Autodesk Inventor part; units mm, degrees
ref_plane "YZ Plane" through (0, 0, 0) normal (1, 0, 0) x (0, 1, 0)
ref_plane "XZ Plane" through (0, 0, 0) normal (0, 1, 0) x (-1, 0, 0)
ref_plane "XY Plane" through (0, 0, 0) normal (0, 0, 1) x (1, 0, 0)
sketch "Sketch1" plane through (0, 0, 0) normal (0, 0, 1) x (1, 0, 0)
  line L0 (0, 0) -> (-140, 0)
  line L1 (-140, 0) -> (-140, 140)
  line L2 (-140, 140) -> (0, 140)
  line L3 (0, 140) -> (0, 0)
  circle A0 centre (-70, 70) radius 14.35
  line L4 (-130, 124.4) -> (-130, 130)
  line L5 (-10, 124.4) -> (-10, 130)
  line L6 (-10, 15.6) -> (-10, 10)
  line L7 (-130, 15.6) -> (-130, 10)
  line L8 (-140, 140) -> (-110, 140)
  line L9 (-110.0005, 135.0005) -> (-110.0005, 113.536)
  line L10 (-113.536, 110) -> (-135, 110)
  line L11 (-140, 110) -> (-140, 140)
  line L12 (-140, 0) -> (-110, 0)
  line L13 (-109.9998, 5.0002) -> (-109.9998, 26.4642)
  line L14 (-113.536, 30) -> (-135, 30)
  line L15 (-140, 30) -> (-140, 0)
  line L16 (0, 0) -> (-30, 0)
  line L17 (-30, 5.0002) -> (-30, 26.464)
  line L18 (-26.4645, 30) -> (-5, 30)
  line L19 (0, 30) -> (0, 0)
  line L20 (0, 140) -> (-30, 140)
  line L21 (-30, 135.0005) -> (-30, 113.536)
  line L22 (-26.4638, 110.0002) -> (-5, 110.0002)
  line L23 (0, 110) -> (0, 140)
  line L24 (-110.0005, 113.536) -> (-80.0116, 83.5551)
  line L25 (-56.4494, 59.9849) -> (-26.4645, 30)
  line L26 (-113.536, 110) -> (-83.5508, 80.0148)
  line L27 (-59.9852, 56.4492) -> (-30, 26.464)
  line L28 (-113.536, 30) -> (-83.5508, 59.9852)
  line L29 (-59.9861, 83.5534) -> (-29.9997, 113.5363)
  line L30 (-109.9998, 26.4642) -> (-80.0148, 56.4492)
  line L31 (-56.4492, 80.0148) -> (-26.4638, 110.0002)
  line L32 (-135, 110) -> (-135, 30)
  line L33 (-140, 30) -> (-140, 110)
  line L34 (-5, 110.0002) -> (-5, 30)
  line L35 (0, 30) -> (0, 110)
  line L36 (-110, 140) -> (-30, 140)
  line L37 (-30, 135.0005) -> (-110.0005, 135.0005)
  line L38 (-30, 0) -> (-110, 0)
  line L39 (-109.9998, 5.0002) -> (-30, 5.0002)
  arc A1 (-83.5508, 80.0148) -> (-83.5508, 59.9852) centre (-70, 70) ccw
  arc A2 (-59.9861, 83.5534) -> (-80.0116, 83.5551) centre (-70, 70) ccw
  arc A3 (-80.0148, 56.4492) -> (-59.9852, 56.4492) centre (-70, 70) ccw
  arc A4 (-56.4494, 59.9849) -> (-56.4492, 80.0148) centre (-70, 70) ccw
  line L40 (-130, 130) -> (-124.4, 130)
  line L41 (-124.4, 130) -> (-124.4, 119.4)
  line L42 (-124.4, 119.4) -> (-130, 119.4)
  line L43 (-130, 119.4) -> (-130, 130)
  line L44 (-130, 10) -> (-124.4, 10)
  line L45 (-124.4, 10) -> (-124.4, 20.6)
  line L46 (-124.4, 20.6) -> (-130, 20.6)
  line L47 (-130, 20.6) -> (-130, 10)
  line L48 (-10, 10) -> (-15.6, 10)
  line L49 (-15.6, 10) -> (-15.6, 20.6)
  line L50 (-15.6, 20.6) -> (-10, 20.6)
  line L51 (-10, 20.6) -> (-10, 10)
  line L52 (-10, 130) -> (-15.6, 130)
  line L53 (-15.6, 130) -> (-15.6, 119.4)
  line L54 (-15.6, 119.4) -> (-10, 119.4)
  line L55 (-10, 119.4) -> (-10, 130)
  line L56 (-113.536, 30) -> (-109.9998, 26.4642)
  line L57 (-30, 26.464) -> (-26.4645, 30)
  line L58 (-30, 113.536) -> (-26.4638, 110.0002)
  line L59 (-110.0005, 113.536) -> (-113.536, 110)
  point P0 (-110, 113.5355)
  point P1 (-110, 26.464)
  point P2 (-26.464, 110)
extrude "Extrusion2" add sketch "Sketch1" along normal blind 5 contours L0 L1 L2 L3 | L24 A2 L29 L58 L31 A4 L25 L57 L27 A3 L30 L56 L28 A1 L26 L59
properties part number "Joints_Remake_TestFit_V1"
Read the model definition and answer for the solid it produces. Units are mm, in the model's axes. Round coordinates to 2 decimals unless told otherwise and drop trailing zeros. Write each loop counter-clockwise with the first axis right and the second up, starting at its lowest first coordinate (ties: lowest second). Pieces come first, ordered by that corner, then holes.
1. The part is cut by section B-B, the plane y = 115.5. Determine the outline of the cut face in (x, z), then the cut area to 3 significant figures.
2. Determine the mould class of faces 1 (the face through (-15.6, 15, 2)), 2 (the face through (-69, 0, 2)) for opening direction Y: pulls with the +Y half, pulls with the -Y half, needs draft (parallel to the pull), parting line crosses it, or undercut.
3. Straight lines are drawn through the part: L1, parallel to Y at x = -70, z = 1.2; L2, parallel to X at y = 70.5, z = 3.7; L3, parallel to X at y = 104.5, z = 1.55. For each, find the intervals that lie inside material, in ascending order.
4. The part is cut by section C-C, the plane x = -70. Determine the outline of the cut face in (y, z).
5. The part is cut by section D-D, the plane z = 1.85. State how many separate pieces and enclosed holes the cut face has, then the cut area to 3 significant figures.
6. The part is cut by section A-A, the plane y = 70. Determine the outline of the cut face in (x, z), then the cut area to 3 significant figures.
Values:
1. outline: (-140, 0) - (-110, 0) - (-110, 5) - (-140, 5) - close; (-30, 0) - (0, 0) - (0, 5) - (-30, 5) - close
1. area: 300 mm2
2. face 1: undercut
2. face 2: pulls with the -Y half
3. L1: y = 0 to 5, 53.15 to 55.65, 84.35 to 86.85, 135 to 140
3. L2: x = -140 to -135, -86.84 to -84.34, -55.66 to -53.16, -5 to 0
3. L3: x = -140 to -135, -108.04 to -100.96, -39.04 to -31.96, -5 to 0
4. outline: (0, 0) - (5, 0) - (5, 5) - (0, 5) - close; (53.15, 0) - (55.65, 0) - (55.65, 5) - (53.15, 5) - close; (84.35, 0) - (86.85, 0) - (86.85, 5) - (84.35, 5) - close; (135, 0) - (140, 0) - (140, 5) - (135, 5) - close
5. separate pieces: 1
5. enclosed holes: 9
5. area: 6,030 mm2
6. outline: (-140, 0) - (-135, 0) - (-135, 5) - (-140, 5) - close; (-86.85, 0) - (-84.35, 0) - (-84.35, 5) - (-86.85, 5) - close; (-55.65, 0) - (-53.15, 0) - (-53.15, 5) - (-55.65, 5) - close; (-5, 0) - (0, 0) - (0, 5) - (-5, 5) - close
6. area: 75.0 mm2
